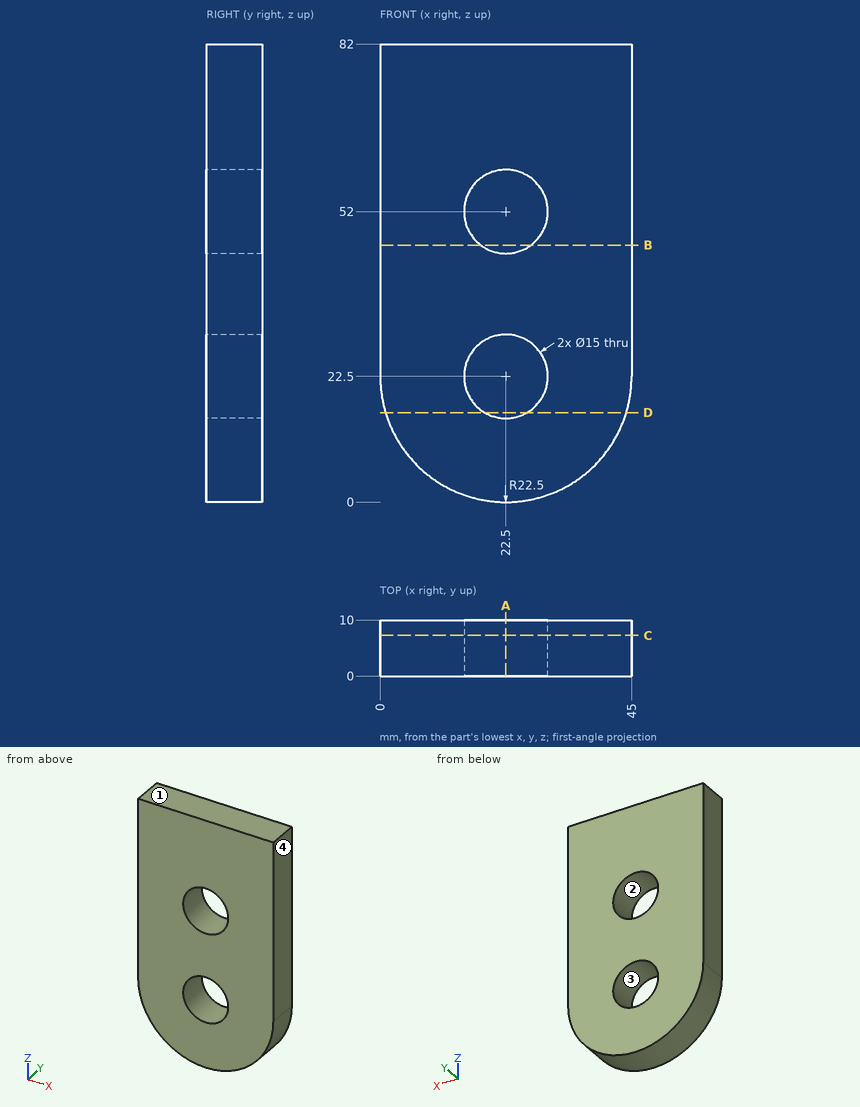
Check sheet for the drawn part. Datum: minimum x, y, z corner. Units: mm. Round coordinates to 2 decimals unless told otherwise and drop trailing zeros. Write each loop counter-clockwise with the first axis right and the second up, starting at its lowest first coordinate (ties: lowest second). Pieces come first, ordered by that corner, then holes. Notation, with made-up numbers: (65, 23.25) - (105, 23.25) arc R22 ccw to (105, 50.25) - close; hole circle Ø9 at (-16.5, 10.25). An arc over 180 degrees is marked (long way). Return JSON: item names as keys, results as strings.
Q1. Cross-section at B-B (z = 46). Record the boundary of the cut face in (x, y), then the cut area to 3 significant figures.
Returned:
{"outline": "(0, 0) - (18, 0) - (18, 10) - (0, 10) - close; (27, 0) - (45, 0) - (45, 10) - (27, 10) - close", "area": "360 mm²"}
Q2. Depth check by flat-ended pin: P1, Ø3, axis at y = 4.5, z = 66.5, coming from the -X side. Enter the tip coordinate at first touch or a pass-through.
Returned:
{"P1": "stops at x = 0"}
Q3. Scan lines: L1, parallel to Z at x = 22.5, y = 2.5; L2, parallel to Z at x = 19, y = 3; L3, parallel to X at y = 2.25, z = 52.5. Record each from-to range of solid material in increasing order. Write a range as from..to.
Returned:
{"L1": "z = 0..15, 30..44.5, 59.5..82", "L2": "z = 0.27..15.87, 29.13..45.37, 58.63..82", "L3": "x = 0..15.02, 29.98..45"}
Q4. Cross-section at C-C (y = 7.25). Record the boundary of the cut face in (x, z), then the cut area to 3 significant figures.
Returned:
{"outline": "(0, 22.5) arc R22.5 ccw to (45, 22.5) - (45, 82) - (0, 82) - close; hole circle Ø15 at (22.5, 22.5); hole circle Ø15 at (22.5, 52)", "area": "3,120 mm²"}
Q5. Cross-section at A-A (x = 22.5). Record the boundary of the cut face in (y, z), then the cut area to 3 significant figures.
Returned:
{"outline": "(0, 0) - (10, 0) - (10, 15) - (0, 15) - close; (0, 30) - (10, 30) - (10, 44.5) - (0, 44.5) - close; (0, 59.5) - (10, 59.5) - (10, 82) - (0, 82) - close", "area": "520 mm²"}
Q6. Cross-section at D-D (z = 16). Record the boundary of the cut face in (x, y), then the cut area to 3 significant figures.
Returned:
{"outline": "(0.96, 0) - (18.76, 0) - (18.76, 10) - (0.96, 10) - close; (26.24, 0) - (44.04, 0) - (44.04, 10) - (26.24, 10) - close", "area": "356 mm²"}
Q7. Draft check along X on the marked faces 1, 2, 3 and 4. Enter one of: released by +X, released by -X, zero draft, split by the parting line, or undercut.
Returned:
{"face 1": "zero draft", "face 2": "undercut", "face 3": "undercut", "face 4": "released by +X"}
